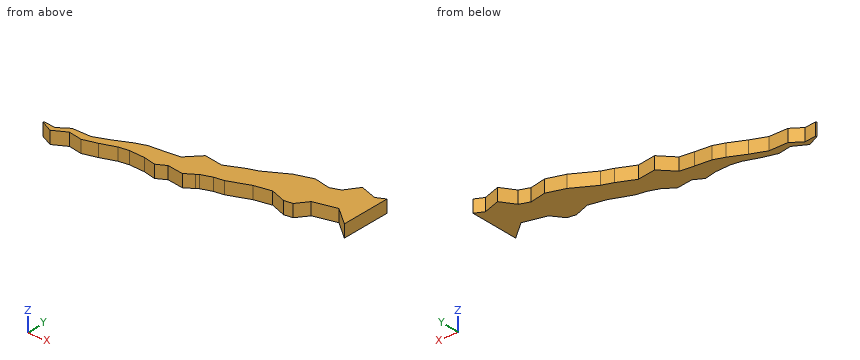
```python
from build123d import *

# Parameters (mm, degrees)
AUFSATZ_LINEAR_AUSTRAGEN1_DEPTH = 3


with BuildPart() as part:
    # Model → Aufsatz-Linear austragen1 (new body)
    with BuildSketch(Plane.XY):
        Polygon((65.064121, 21.807638525), (62.991032211, 20.74255457), (58.984084126, 22.00272439), (56.803026288, 18.838800991), (54.47947364, 17.944388553), (50.590045168, 18.671312469), (46.453572189, 17.279002848), (41.134110077, 14.142873543), (38.589728344, 13.192799771), (34.5476256, 11.233834156), (30.138450774, 11.805962104), (27.107969747, 8.540929476), (23.780046409, 8.100068659), (19.936127337, 7.664785218), (17.41204954, 6.721746516), (13.666478399, 4.851440527), (10.094159276, 3.31838703), (5.581557396, 3.252404134), (3.018679888, 1.437790494), (0.267615815, 1.681687606), (0.139255665, 1.450037519), (2.981259215, 0.112718703), (6.103803639, 1.911841244), (9.316252445, 1.390545324), (12.654979952, 2.375260761), (16.2205293, 3.716688419), (18.59217244, 4.136227412), (22.278782524, 4.040377998), (25.178549561, 3.451362989), (27.378100316, 4.707930745), (31.154159786, 4.275156188), (33.120124598, 5.602792152), (33.743945474, 6.05917628), (36.273485131, 6.993163334), (38.623931318, 7.409502482), (43.568119128, 9.480736692), (47.587851937, 10.360104548), (51.289746217, 9.100216289), (53.306429565, 9.430364623), (55.321012546, 12.093179433), (60.7300212, 13.5422604), (65.064121, 10.068977561), align=None)
    extrude(amount=AUFSATZ_LINEAR_AUSTRAGEN1_DEPTH)


solid = part.part
```
Verification items for the finished model (mm, model axes). Give positions to 0.01 mm unless a question says otherwise; leave off trailing zeros. Order: outer loops, then holes, each group sorted by start corner. A loop starts at its lowest first (then second) coordinate and runs counter-clockwise, first axis right, second up. Notation, with made-up numbers: M 23,31 L 40,31 A8 cw 40,44 Z; hole C 88,89.25 d7. An arc over 180 degrees is marked long. Return JSON: item names as keys, results as strings. Group by question number.
1) Section check A-A on x = 20.5. Record the cut outline in (y, z).
2) Section check B-B on y = 20. Record the cut outline in (x, z), and give its area (3 significant figures).
3) Go/stop test with flat-tipped pins: pin 1 Ø1.5 at (x, z) = (21.5, 1.5) entering from +Y; pin 2 Ø1 at (y, z) = (9.5, 0.5) entering from -X. Record where each tip stops, or that it passes through.
4) Scan lines: line 1 (X direction, y = 14.25, z = 2.6); line 2 (Y direction, x = 23.5, z = 0.2); line 3 (X direction, y = 12, z = 0.9). Record each from-to range of solid material in increasing order.
Answer block:
{
 "1": {"outline": "M 4.09,0 L 7.73,0 L 7.73,3 L 4.09,3 Z"},
 "2": {"outline": "M 57.6,0 L 65.06,0 L 65.06,3 L 57.6,3 Z", "area": "22.4 mm^2"},
 "3": {"pin 1": "stops at y = 7.93", "pin 2": "stops at x = 27.53"},
 "4": {"line 1": "x = 41.32 to 65.06", "line 2": "y = 3.79 to 8.07", "line 3": "x = 36.13 to 55.25, 62.65 to 65.06"}
}
